from build123d import *

# Parameters (mm, degrees)
SKETCH_1_W          = 40
SKETCH_1_H          = 40
EXTRUDE_1_DEPTH     = 550
CUT_EXTRUDE_1_REACH = 558.07
SKETCH_2_R          = 3.5
SKETCH_2_R_2        = 3
FILLET_1_R          = 5


with BuildPart() as part:
    # 草图1 → 凸台-拉伸1 (new body)
    with BuildSketch(Plane(origin=(0, 0, 0), x_dir=(0, 0, -1), z_dir=(1, 0, 0))):
        with Locations((40.704960836, 35.035758607)):
            Rectangle(SKETCH_1_W, SKETCH_1_H)
    extrude(amount=EXTRUDE_1_DEPTH)

    # 草图2 → 切除-拉伸1 (cut, up to next)
    with BuildSketch(Plane(origin=(550, 0, 0), x_dir=(0, 0, -1), z_dir=(1, 0, 0)), mode=Mode.PRIVATE) as cut_extrude_1_sk1:
        with Locations((40.704960836, 35.035758607)):
            Circle(SKETCH_2_R)
    cut_extrude_1_tool1 = extrude(cut_extrude_1_sk1.sketch, amount=-CUT_EXTRUDE_1_REACH, mode=Mode.PRIVATE) & part.part
    # 草图2 → 切除-拉伸1 (cut, up to next)
    with BuildSketch(Plane(origin=(550, 0, 0), x_dir=(0, 0, -1), z_dir=(1, 0, 0)), mode=Mode.PRIVATE) as cut_extrude_1_sk2:
        with Locations((25.854960836, 49.885758607)):
            Circle(SKETCH_2_R_2)
    cut_extrude_1_tool2 = extrude(cut_extrude_1_sk2.sketch, amount=-CUT_EXTRUDE_1_REACH, mode=Mode.PRIVATE) & part.part
    # 草图2 → 切除-拉伸1 (cut, up to next)
    with BuildSketch(Plane(origin=(550, 0, 0), x_dir=(0, 0, -1), z_dir=(1, 0, 0)), mode=Mode.PRIVATE) as cut_extrude_1_sk3:
        with Locations((25.854960836, 20.185758607)):
            Circle(SKETCH_2_R_2)
    cut_extrude_1_tool3 = extrude(cut_extrude_1_sk3.sketch, amount=-CUT_EXTRUDE_1_REACH, mode=Mode.PRIVATE) & part.part
    # 草图2 → 切除-拉伸1 (cut, up to next)
    with BuildSketch(Plane(origin=(550, 0, 0), x_dir=(0, 0, -1), z_dir=(1, 0, 0)), mode=Mode.PRIVATE) as cut_extrude_1_sk4:
        with Locations((55.554960836, 49.885758607)):
            Circle(SKETCH_2_R_2)
    cut_extrude_1_tool4 = extrude(cut_extrude_1_sk4.sketch, amount=-CUT_EXTRUDE_1_REACH, mode=Mode.PRIVATE) & part.part
    # 草图2 → 切除-拉伸1 (cut, up to next)
    with BuildSketch(Plane(origin=(550, 0, 0), x_dir=(0, 0, -1), z_dir=(1, 0, 0)), mode=Mode.PRIVATE) as cut_extrude_1_sk5:
        with Locations((55.554960836, 20.185758607)):
            Circle(SKETCH_2_R_2)
    cut_extrude_1_tool5 = extrude(cut_extrude_1_sk5.sketch, amount=-CUT_EXTRUDE_1_REACH, mode=Mode.PRIVATE) & part.part
    # 草图2 → 切除-拉伸1 (cut, up to next)
    with BuildSketch(Plane(origin=(550, 0, 0), x_dir=(0, 0, -1), z_dir=(1, 0, 0)), mode=Mode.PRIVATE) as cut_extrude_1_sk6:
        Polygon((36.704960836, 15.035758607), (36.704960836, 19.535758607), (34.004960836, 19.535758607), (34.004960836, 17.735758607), (31.004960836, 17.735758607), (31.004960836, 22.235758607), (35.704960836, 27.275758607), (45.704960836, 27.275758607), (50.404960836, 22.235758607), (50.404960836, 17.735758607), (47.404960836, 17.735758607), (47.404960836, 19.535758607), (44.704960836, 19.535758607), (44.704960836, 15.035758607), align=None)
    cut_extrude_1_tool6 = extrude(cut_extrude_1_sk6.sketch, amount=-CUT_EXTRUDE_1_REACH, mode=Mode.PRIVATE) & part.part
    # 草图2 → 切除-拉伸1 (cut, up to next)
    with BuildSketch(Plane(origin=(550, 0, 0), x_dir=(0, 0, -1), z_dir=(1, 0, 0)), mode=Mode.PRIVATE) as cut_extrude_1_sk7:
        Polygon((44.704960836, 55.035758607), (44.704960836, 50.535758607), (47.404960836, 50.535758607), (47.404960836, 52.335758607), (50.404960836, 52.335758607), (50.404960836, 47.835758607), (45.704960836, 42.795758607), (35.704960836, 42.795758607), (31.004960836, 47.835758607), (31.004960836, 52.335758607), (34.004960836, 52.335758607), (34.004960836, 50.535758607), (36.704960836, 50.535758607), (36.704960836, 55.035758607), align=None)
    cut_extrude_1_tool7 = extrude(cut_extrude_1_sk7.sketch, amount=-CUT_EXTRUDE_1_REACH, mode=Mode.PRIVATE) & part.part
    # 草图2 → 切除-拉伸1 (cut, up to next)
    with BuildSketch(Plane(origin=(550, 0, 0), x_dir=(0, 0, -1), z_dir=(1, 0, 0)), mode=Mode.PRIVATE) as cut_extrude_1_sk8:
        Polygon((20.704960836, 31.035758607), (20.704960836, 39.035758607), (25.204960836, 39.035758607), (25.204960836, 41.735758607), (23.404960836, 41.735758607), (23.404960836, 44.735758607), (27.954960836, 44.735758607), (32.944960836, 40.035758607), (32.944960836, 30.035758607), (27.954960836, 25.335758607), (23.404960836, 25.335758607), (23.404960836, 28.335758607), (25.204960836, 28.335758607), (25.204960836, 31.035758607), align=None)
    cut_extrude_1_tool8 = extrude(cut_extrude_1_sk8.sketch, amount=-CUT_EXTRUDE_1_REACH, mode=Mode.PRIVATE) & part.part
    # 草图2 → 切除-拉伸1 (cut, up to next)
    with BuildSketch(Plane(origin=(550, 0, 0), x_dir=(0, 0, -1), z_dir=(1, 0, 0)), mode=Mode.PRIVATE) as cut_extrude_1_sk9:
        Polygon((60.704960836, 31.035758607), (56.204960836, 31.035758607), (56.204960836, 28.335758607), (58.004960836, 28.335758607), (58.004960836, 25.335758607), (53.454960836, 25.335758607), (48.464960836, 30.035758607), (48.464960836, 40.035758607), (53.454960836, 44.735758607), (58.004960836, 44.735758607), (58.004960836, 41.735758607), (56.204960836, 41.735758607), (56.204960836, 39.035758607), (60.704960836, 39.035758607), align=None)
    cut_extrude_1_tool9 = extrude(cut_extrude_1_sk9.sketch, amount=-CUT_EXTRUDE_1_REACH, mode=Mode.PRIVATE) & part.part
    add(cut_extrude_1_tool1.solids().sort_by_distance((550, 35.035759, -40.704961))[0], mode=Mode.SUBTRACT)
    add(cut_extrude_1_tool2.solids().sort_by_distance((550, 49.885759, -25.854961))[0], mode=Mode.SUBTRACT)
    add(cut_extrude_1_tool3.solids().sort_by_distance((550, 20.185759, -25.854961))[0], mode=Mode.SUBTRACT)
    add(cut_extrude_1_tool4.solids().sort_by_distance((550, 49.885759, -55.554961))[0], mode=Mode.SUBTRACT)
    add(cut_extrude_1_tool5.solids().sort_by_distance((550, 20.185759, -55.554961))[0], mode=Mode.SUBTRACT)
    add(cut_extrude_1_tool6.solids().sort_by_distance((550, 21.537481, -40.704961))[0], mode=Mode.SUBTRACT)
    add(cut_extrude_1_tool7.solids().sort_by_distance((550, 48.534036, -40.704961))[0], mode=Mode.SUBTRACT)
    add(cut_extrude_1_tool8.solids().sort_by_distance((550, 35.035759, -27.209927))[0], mode=Mode.SUBTRACT)
    add(cut_extrude_1_tool9.solids().sort_by_distance((550, 35.035759, -54.199995))[0], mode=Mode.SUBTRACT)

    # 圆角1
    fillet_1_edges = [part.edges().sort_by_distance(p)[0] for p in [
        (275, 55.035758607, -20.704960836),
        (275, 55.035758607, -60.704960836),
        (275, 15.035758607, -60.704960836),
        (275, 15.035758607, -20.704960836),
    ]]
    fillet(fillet_1_edges, radius=FILLET_1_R)


solid = part.part
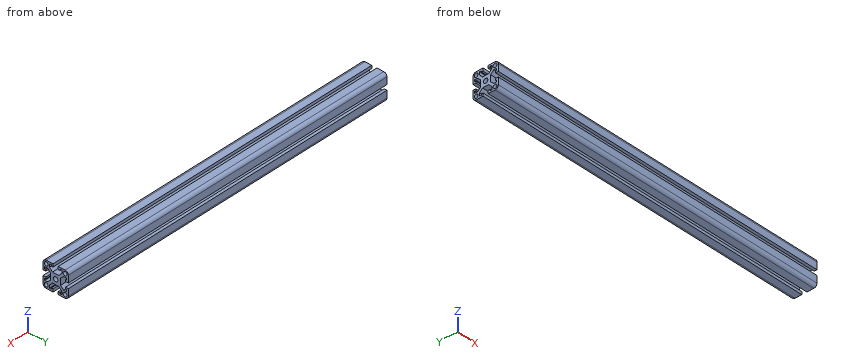
Could you check a few things on this model? Use its own coordinates, in mm. Round coordinates to 2 decimals unless told otherwise and drop trailing zeros.
Q1. Imagine slicing it at A-A, the plane x = 95.5. State how many separate pieces and enclosed holes the cut face has, then the cut area to 3 significant figures.
Geometry says:
separate pieces: 1
enclosed holes: 5
area: 733 mm2
Q2. Please list where these lines run through material, in increasing order: probe 1 along Y at (x, z) = (324, -45.5); probe 2 along Z at (x, y) = (468, 19.5); probe 3 along Z at (x, y) = (79, 49.5).
Geometry says:
probe 1: y = 15.04 to 19.54, 27.28 to 42.8, 50.54 to 55.04
probe 2: z = -60.68 to -58.48, -52.63 to -50.4, -47.4 to -44.7, -36.7 to -34, -31 to -28.78, -22.93 to -20.73
probe 3: z = -60.7 to -58.53, -52.58 to -50.4, -31 to -28.83, -22.88 to -20.7
Q3. I'm going to push flat-ended pins straight in: P1, Ø1.5, axis at y = 20, z = -44, coming from the +X side; P2, Ø3.5, axis at x = 211.5, y = 17, coming from the +Z side; P3, Ø2, axis at x = 399, z = -24, coming from the +Y side; P4, Ø2, axis at x = 254.5, z = -23, coming from the +Y side. Where does each tip first touch, or does it pass through?
Geometry says:
P1: passes through
P2: stops at z = -20.87
P3: stops at y = 54.99
P4: stops at y = 54.74
